from build123d import *

# Parameters (mm, degrees)
SKETCH_3_R           = 14.347327659
SKETCH_3_W           = 19
SKETCH_3_H           = 19
CUT_EXTRUDE_1_DEPTH  = 15
SKETCH_4_R           = 9.80838312
CUT_EXTRUDE_2_DEPTH  = 4
SKETCH_5_R           = 11.664818178
CUT_EXTRUDE_3_DEPTH  = 2.424756107
SKETCH_6_R           = 18.248215306
SKETCH_6_W           = 19
SKETCH_6_H           = 19
CUT_EXTRUDE_4_DEPTH  = 3
EXTRUDE_1_DEPTH      = 17
EXTRUDE_1_DEPTH_BACK = 47
SKETCH_8_R           = 4.5
SKETCH_9_R           = 5.7
EXTRUDE_2_DEPTH      = 8
EXTRUDE_3_DEPTH      = 32
EXTRUDE_3_DEPTH_BACK = 32
SKETCH_10_R          = 4.5


with BuildPart() as part:
    # Sketch 2 → Revolve 1 (revolve)
    with BuildSketch(Plane.XY, mode=Mode.PRIVATE) as revolve_1_sk:
        Polygon((0, 110), (12.5, 110), (12.5, 62), (15, 62), (15, 40), (10, 40), (10, 30), (10.5, 30), (10.5, 27.575243893), (6.508274003, 27.575243893), (6.508274003, 24), (9, 24), (9, 20), (5.5, 20), (5.5, 0), (0, 0), align=None)
    revolve(revolve_1_sk.sketch.rotate(Axis((0, 0, 0), (0, 1, 0)), 90), axis=Axis((0, 0, 0), (0, 1, 0)))

    # Sketch 3 → Cut-Extrude 1 (cut)
    with BuildSketch(Plane(origin=(0, 110, 0), x_dir=(1, 0, 0), z_dir=(0, 1, 0))):
        Circle(SKETCH_3_R)
        Rectangle(SKETCH_3_W, SKETCH_3_H, mode=Mode.SUBTRACT)
    extrude(amount=-CUT_EXTRUDE_1_DEPTH, mode=Mode.SUBTRACT)

    # Sketch 4 → Cut-Extrude 2 (cut)
    with BuildSketch(Plane.XZ.offset(-20)):
        Circle(SKETCH_4_R)
        Polygon((0, 9), (-7.794228634, 4.5), (-7.794228634, -4.5), (0, -9), (7.794228634, -4.5), (7.794228634, 4.5), align=None, mode=Mode.SUBTRACT)
    extrude(amount=-CUT_EXTRUDE_2_DEPTH, mode=Mode.SUBTRACT)

    # Sketch 5 → Cut-Extrude 3 (cut)
    with BuildSketch(Plane.XZ.offset(-27.575243893)):
        Circle(SKETCH_5_R)
        Polygon((0, 10.5), (-9.09326674, 5.25), (-9.09326674, -5.25), (0, -10.5), (9.09326674, -5.25), (9.09326674, 5.25), align=None, mode=Mode.SUBTRACT)
    extrude(amount=-CUT_EXTRUDE_3_DEPTH, mode=Mode.SUBTRACT)

    # Sketch 6 → Cut-Extrude 4 (cut)
    with BuildSketch(Plane.XZ.offset(-40)):
        Circle(SKETCH_6_R)
        Rectangle(SKETCH_6_W, SKETCH_6_H, mode=Mode.SUBTRACT)
    extrude(amount=-CUT_EXTRUDE_4_DEPTH, mode=Mode.SUBTRACT)

    # Sketch 9 → Extrude 2 (add)
    with BuildSketch(Plane(origin=(0, 110, 0), x_dir=(1, 0, 0), z_dir=(0, 1, 0))):
        with Locations(Location((0, 0, 0), (0, 0, 270))):
            Circle(SKETCH_9_R)
    extrude(amount=EXTRUDE_2_DEPTH)



with BuildPart() as body_2:
    # Sketch 8 → Extrude 1 (new, two sides: drawn at the far end of the back side and taken through both)
    with BuildSketch(Plane.XY.offset(15).offset(-EXTRUDE_1_DEPTH_BACK)):
        with Locations((0, 54.5)):
            Circle(SKETCH_8_R)
    extrude(amount=EXTRUDE_1_DEPTH + EXTRUDE_1_DEPTH_BACK)


with BuildPart() as part_1:
    add(part.part)

    add(body_2.part)  # Extrude 3 merges body 2
    # Sketch 10 → Extrude 3 (add, two sides: drawn at the far end of the back side and taken through both)
    with BuildSketch(Plane(origin=(0, 0, 0), x_dir=(0, 0, -1), z_dir=(1, 0, 0)).offset(-EXTRUDE_3_DEPTH_BACK)):
        with Locations((0, 54.5)):
            Circle(SKETCH_10_R)
    extrude(amount=EXTRUDE_3_DEPTH + EXTRUDE_3_DEPTH_BACK)


solid = part_1.part
Part model, mm, in its own coordinate system. A direction names the side the tool comes from. Give positions to 0.01 mm unless a question says otherwise; leave off trailing zeros. Loops run counter-clockwise (first coordinate to the right, second up) from the corner with the lowest first, then second, coordinate; pieces in that order, holes last. Notation, with made-up numbers: M 74.5,66 L 121.5,66 A34 ccw 121.5,98 Z; hole C 0,-18 d5. An arc over 180 degrees is marked long. Put each result on its own line as item: value. Start each with the question number.
1) 3-axis set-ups, long thin cutter, end or side, ignore diameter. For faces 1 (the flat face through (4.5, 28.8, -7.9)), 2 (the cylindrical face through (23.02, 50.11, 0.98)), 3 (the flat face through (0, 41, -9.5)), 4 (the flat face through (11, 95, 0)), 5 (the cylindrical face through (-8.45, 80.33, 9.21)): which of +Z, -Z, +X, -X, +Y, -Y reach the whole face in a straight line?
2) Saw through at A-A (x = 25). List the corners of the cut face in (y, z).
3) Probe probe 1 along Z at (x, y) = (0.5, 102); probe 2 along Y at (x, z) = (0.5, -13); probe 3 along X at (y, z) = (110.5, -0.5). List the from-to ranges inside material, lowest first.
4) Flat gauge pins, fed straight in: pin 1 (2.5 mm diameter, centred on x = -3.5, z = -11.5, fed in from +Y); pin 2 (2 mm diameter, centred on x = -6, z = -8.5, fed in from -Y); pin 3 (1.5 mm diameter, centred on x = 0.5, z = 15.5, fed in from -Y). Where does each tip first touch, or does it go through?
5) Saw through at B-B (y = 92.5). List the corners of the cut face in (x, z), then the cut area to 3 significant figures.
Numbers:
1. face 1: -Z, +X, -Y
1. face 2: +X
1. face 3: -Z, +X, -X
1. face 4: +Z, -Z, +X, +Y
1. face 5: +Y
2. outline: C 54.5,0 d9
3. probe 1: -9.5 to 9.5
3. probe 2: 43 to 62
3. probe 3: -5.68 to 5.68
4. pin 1: y = 95
4. pin 2: y = 30
4. pin 3: y = 43
5. outline: C 0,0 d25
5. area: 491 mm^2
